Geometry: final body of the model. Coordinates: model frame, mm. Face numbers are marked on the shaded views. A direction names the side the tool comes from. Round coordinates to 2 decimals unless told otherwise and drop trailing zeros. Write each loop counter-clockwise with the first axis right and the second up, starting at its lowest first coordinate (ties: lowest second). Pieces come first, ordered by that corner, then holes. Notation, with made-up numbers: M 65.25,-11 L 98.25,-11 A28 cw 98.25,21 Z; hole C 4.25,38 d1. An arc over 180 degrees is marked long. Put each result on its own line as item: value. Start each with the question number.
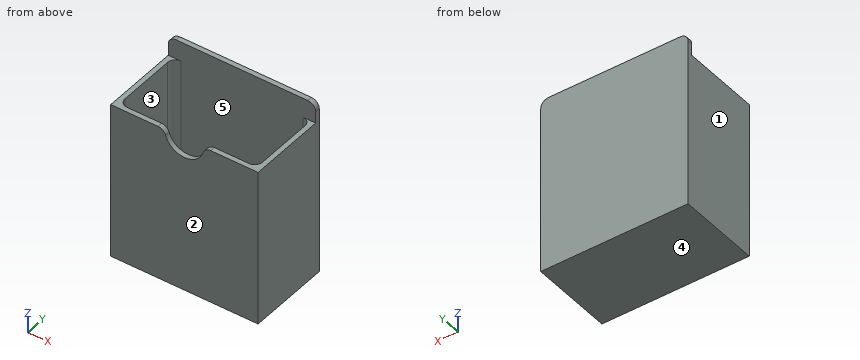
```python
from build123d import *

# Parameters (mm, degrees)
F0_W     = 95.25
F0_H     = 53.975
F1_DEPTH = 2.032
F2_W     = 95.25
F2_H     = 53.975
F2_W_2   = 88.9
F2_H_2   = 47.625
F3_DEPTH = 99.568
F4_W     = 95.25
F4_H     = 3.175
F5_DEPTH = 12.7
F6_R     = 5.08
F7_R     = 5.08
F8_R     = 12.7
F9_DEPTH = 6.35
F10_R    = 5.08


with BuildPart() as f1:
    # F0 (on Top) → F1 (new body)
    with BuildSketch(Plane.XY):
        with Locations((47.625, 26.9875)):
            Rectangle(F0_W, F0_H)
    extrude(amount=F1_DEPTH)

    # F2 (on face) → F3 (join)
    with BuildSketch(Plane.XY.offset(2.032)):
        with Locations((47.625, 26.9875)):
            Rectangle(F2_W, F2_H)
        with Locations((47.625, 26.9875)):
            Rectangle(F2_W_2, F2_H_2, mode=Mode.SUBTRACT)
    extrude(amount=F3_DEPTH)

    # F4 (on face) → F5 (join)
    with BuildSketch(Plane.XY.offset(101.6)):
        with Locations((47.625, 52.3875)):
            Rectangle(F4_W, F4_H)
    extrude(amount=F5_DEPTH)

    # F6
    f6_edges = [f1.edges().sort_by_distance(p)[0] for p in [
        (0, 52.3875, 114.3),
        (95.25, 52.3875, 114.3),
    ]]
    fillet(f6_edges, radius=F6_R)

    # F7
    f7_edges = [f1.edges().sort_by_distance(p)[0] for p in [
        (92.075, 50.8, 51.816),
        (3.175, 50.8, 51.816),
        (3.175, 3.175, 51.816),
        (92.075, 3.175, 51.816),
    ]]
    fillet(f7_edges, radius=F7_R)

    # F8 (on face) → F9 (cut)
    with BuildSketch(Plane.XZ):
        with Locations((47.625, 101.6)):
            Circle(F8_R)
    extrude(amount=-F9_DEPTH, mode=Mode.SUBTRACT)

    # F10
    f10_edges = [f1.edges().sort_by_distance(p)[0] for p in [
        (60.325, 1.5875, 101.6),
        (34.925, 1.5875, 101.6),
    ]]
    fillet(f10_edges, radius=F10_R)


solid = f1.part
```
1) First-contact query: pin 1 (2 mm diameter, centred on x = 83, y = 42, fed in from +Z). Flat tip, straight axial feed; report the tip coordinate or a pass-through.
2) Ray query, probe 1 along Y at (x, z) = (19, 15) (3 decimals); probe 2 along X at (y, z) = (8, 81.5); probe 3 along Z at (x, y) = (48, 15). Return the intervals inside material, ascending.
3) Section A-A, the plane z = 29. Output: boundary loops of the cut face in (x, y) (3 decimals).
4) Section C-C, the plane x = 12. Output: boundary loops of the cut face in (y, z) (3 decimals).
5) Access query for the marked faces 4 and 5. Directions: +Z, -Z, +X, -X, +Y, -Y. A direction counts if a zero-diameter tool reaches every point of the face in a straight line with its end or side. Return the directions, or none.
6) Draft query along X for the marked faces 1, 2 and 3. Return one class per face: +X half, -X half, draft (parallel to the pull), parting line (faces both ways), or undercut.
7) Section B-B, the plane y = 22. Output: boundary loops of the cut face in (x, z) (3 decimals), and give its area (3 significant figures).
8) Section D-D, the plane z = 91. Output: boundary loops of the cut face in (x, y) (3 decimals), and give its area (3 significant figures).
Solved:
1. pin 1: stops at z = 2.03
2. probe 1: y = 0 to 3.175, 50.8 to 53.975
2. probe 2: x = 0 to 3.18, 92.07 to 95.25
2. probe 3: z = 0 to 2.03
3. outline: M 0,0 L 95.25,0 L 95.25,53.975 L 0,53.975 Z; hole M 3.175,8.255 A5.08 ccw 8.255,3.175 L 86.995,3.175 A5.08 ccw 92.075,8.255 L 92.075,45.72 A5.08 ccw 86.995,50.8 L 8.255,50.8 A5.08 ccw 3.175,45.72 Z
4. outline: M 0,0 L 53.975,0 L 53.975,114.3 L 50.8,114.3 L 50.8,2.032 L 3.175,2.032 L 3.175,101.6 L 0,101.6 Z
5. face 4: -Z, +X, -X, +Y, -Y
5. face 5: +Z
6. face 1: -X half
6. face 2: draft
6. face 3: undercut
7. outline: M 0,0 L 95.25,0 L 95.25,101.6 L 92.075,101.6 L 92.075,2.032 L 3.175,2.032 L 3.175,101.6 L 0,101.6 Z
7. area: 826 mm2
8. outline: M 0,0 L 40.63,0 L 40.63,3.175 L 8.255,3.175 A5.08 cw 3.175,8.255 L 3.175,45.72 A5.08 cw 8.255,50.8 L 86.995,50.8 A5.08 cw 92.075,45.72 L 92.075,8.255 A5.08 cw 86.995,3.175 L 54.62,3.175 L 54.62,0 L 95.25,0 L 95.25,53.975 L 0,53.975 Z
8. area: 885 mm2
